Design review of the part shown in the three views and the two pictorial views. Dimensions are in mm from the part's minimum x, y and z. Round coordinates to 2 decimals unless told otherwise and drop trailing zeros. Loops run counter-clockwise (first coordinate to the right, second up) from the corner with the lowest first, then second, coordinate; pieces in that order, holes last. Notation, with made-up numbers: M 28,51 L 35,51 A21 ccw 35,82 Z; hole C 38,69 d11. An arc over 180 degrees is marked long. Return JSON: item names as keys, results as strings. Group by question number.
Q1. To check wall thickness, follow line 1 along X through (y, z) = (0.25, 58); line 2 along X through (y, z) = (0.9, 30); line 3 along Z through (x, y) = (43.5, 1.1). State the ranges of each line that lie inside material, in increasing order.
Q2. Consider section B-B (x = 85). State the section outline as (y, z) points.
Q3. Clearance check with flat-ended pins moving along their axes: pin 1 Ø2 at (x, z) = (148.5, 142.5) entering from -Y; pin 2 Ø0.9 at (y, z) = (2, 206) entering from +X; pin 3 Ø0.9 at (x, y) = (43, 2) entering from +Z; pin 4 Ø1.5 at (y, z) = (2.5, 81) entering from -X. State where each tip first meets the part, or that it passes through.
Q4. Consider section A-A (z = 150). State the section outline as (x, y) points.
Q5. Consider section D-D (z = 60). State the section outline as (x, y) points, and give its area (3 significant figures).
Q6. Consider section C-C (y = 1.15). Count the separate pieces of the cut face and the enclosed holes in it, and give its area (3 significant figures).
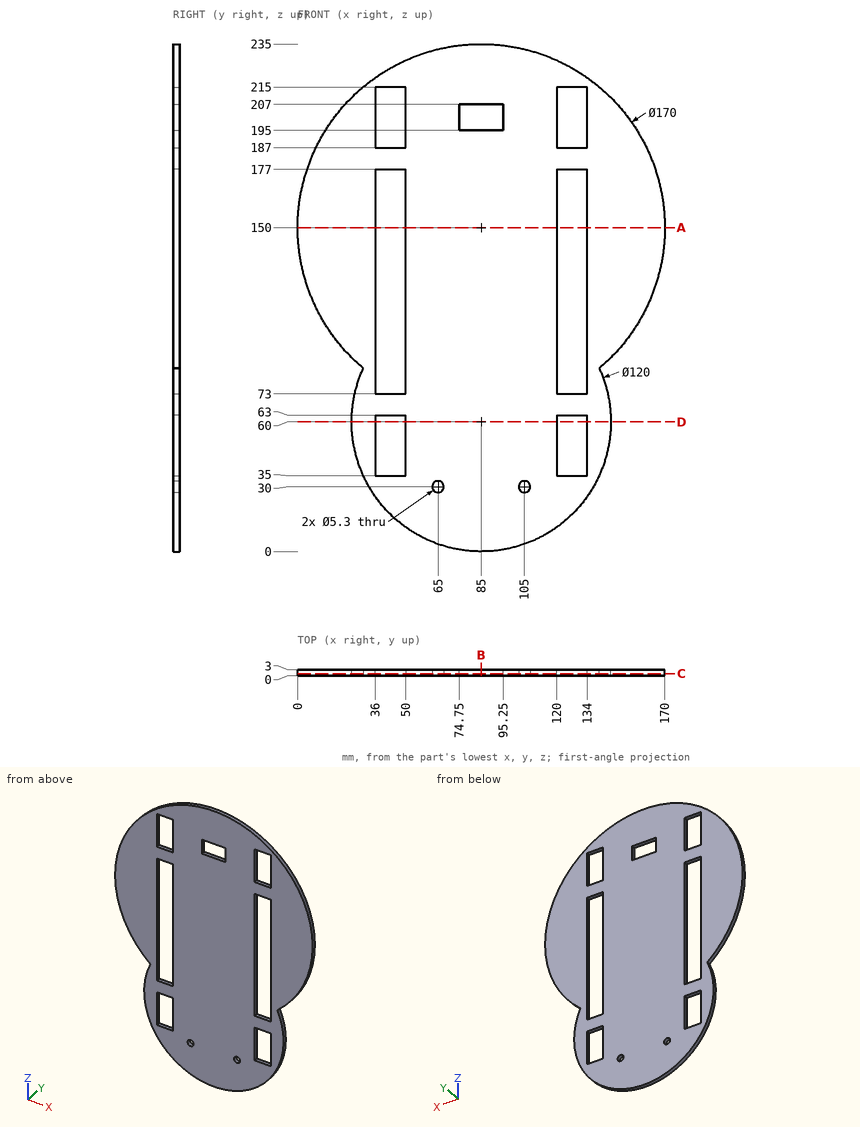
Values:
{
 "1": {"line 1": "x = 25.03 to 36, 50 to 120, 134 to 144.97", "line 2": "x = 33.04 to 62.35, 67.65 to 102.35, 107.65 to 136.96", "line 3": "z = 16.67 to 35, 63 to 73, 177 to 187, 215 to 224.18"},
 "2": {"outline": "M 0,0 L 3,0 L 3,195 L 0,195 Z; M 0,207 L 3,207 L 3,235 L 0,235 Z"},
 "3": {"pin 1": "stops at y = 0", "pin 2": "stops at x = 149.34", "pin 3": "stops at z = 224.15", "pin 4": "stops at x = 28.52"},
 "4": {"outline": "M 0,0 L 36,0 L 36,3 L 0,3 Z; M 50,0 L 120,0 L 120,3 L 50,3 Z; M 134,0 L 170,0 L 170,3 L 134,3 Z"},
 "5": {"outline": "M 25,0 L 36,0 L 36,3 L 25,3 Z; M 50,0 L 120,0 L 120,3 L 50,3 Z; M 134,0 L 145,0 L 145,3 L 134,3 Z", "area": "276 mm2"},
 "6": {"separate pieces": "1", "enclosed holes": "9", "area": "25,000 mm2"}
}
